Part model, mm, in its own coordinate system. Give positions to 0.01 mm unless a question says otherwise; leave off trailing zeros. Write each loop counter-clockwise with the first axis right and the second up, starting at its lowest first coordinate (ties: lowest second). Pieces come first, ordered by that corner, then holes.
```python
from build123d import *

# Parameters (mm, degrees)
SKETCH_1_W           = 0.6
SKETCH_1_H           = 0.6
EXTRUDE_1_DEPTH      = 2
EXTRUDE_2_DEPTH      = 6
EXTRUDE_2_DEPTH_BACK = 5
SKETCH_2_W           = 0.6
SKETCH_2_H           = 0.6


with BuildPart() as part:
    # 草图1 → 凸台-拉伸1 (new body)
    with BuildSketch(Plane.XY):
        Polygon((-0.762, 1.27), (-1.27, 0.762), (-1.27, -0.762), (-0.762, -1.27), (0.762, -1.27), (1.27, -0.762), (1.778, -1.27), (3.302, -1.27), (3.81, -0.762), (4.318, -1.27), (5.842, -1.27), (6.35, -0.762), (6.35, 0.762), (5.842, 1.27), (4.318, 1.27), (3.81, 0.762), (3.302, 1.27), (1.778, 1.27), (1.27, 0.762), (0.762, 1.27), align=None)
        with Locations((2.54, 0)):
            Rectangle(SKETCH_1_W, SKETCH_1_H, mode=Mode.SUBTRACT)
        Rectangle(SKETCH_1_W, SKETCH_1_H, mode=Mode.SUBTRACT)
        with Locations((5.08, 0)):
            Rectangle(SKETCH_1_W, SKETCH_1_H, mode=Mode.SUBTRACT)
    extrude(amount=EXTRUDE_1_DEPTH)

    # 草图2 → 凸台-拉伸2 (add, two sides: drawn at the far end of the back side and taken through both)
    with BuildSketch(Plane.XY.offset(2).offset(-EXTRUDE_2_DEPTH_BACK)):
        Rectangle(SKETCH_2_W, SKETCH_2_H)
        with Locations((2.54, 0)):
            Rectangle(SKETCH_2_W, SKETCH_2_H)
        with Locations((5.08, 0)):
            Rectangle(SKETCH_2_W, SKETCH_2_H)
    extrude(amount=EXTRUDE_2_DEPTH + EXTRUDE_2_DEPTH_BACK)


solid = part.part
```
1) Saw through at A-A, the plane z = 3.5. Write the cut outline in (x, y), then the cut area to 3 significant figures.
Answers follow:
outline: (-0.3, -0.3) - (0.3, -0.3) - (0.3, 0.3) - (-0.3, 0.3) - close; (2.24, -0.3) - (2.84, -0.3) - (2.84, 0.3) - (2.24, 0.3) - close; (4.78, -0.3) - (5.38, -0.3) - (5.38, 0.3) - (4.78, 0.3) - close
area: 1.08 mm2
2) Saw through at C-C, the plane x = 0. Write the cut outline in (y, z), then the cut area to 3 significant figures.
Answers follow:
outline: (-1.27, 0) - (-0.3, 0) - (-0.3, -3) - (0.3, -3) - (0.3, 0) - (1.27, 0) - (1.27, 2) - (0.3, 2) - (0.3, 8) - (-0.3, 8) - (-0.3, 2) - (-1.27, 2) - close
area: 10.5 mm2
3) Wall check: L1, parallel to X at y = 0.1, z = 2.25; L2, parallel to X at y = -1, z = 1.75; L3, parallel to Z at x = 6, y = -0.6. Give the ranges that are in metal, low to high.
Answers follow:
L1: x = -0.3 to 0.3, 2.24 to 2.84, 4.78 to 5.38
L2: x = -1.03 to 1.03, 1.51 to 3.57, 4.05 to 6.11
L3: z = 0 to 2
4) Saw through at D-D, the plane z = 1.5. Write the cut outline in (x, y).
Answers follow:
outline: (-1.27, -0.76) - (-0.76, -1.27) - (0.76, -1.27) - (1.27, -0.76) - (1.78, -1.27) - (3.3, -1.27) - (3.81, -0.76) - (4.32, -1.27) - (5.84, -1.27) - (6.35, -0.76) - (6.35, 0.76) - (5.84, 1.27) - (4.32, 1.27) - (3.81, 0.76) - (3.3, 1.27) - (1.78, 1.27) - (1.27, 0.76) - (0.76, 1.27) - (-0.76, 1.27) - (-1.27, 0.76) - close
5) Saw through at B-B, the plane y = 1.05. Write the cut outline in (x, z), then the cut area to 3 significant figures.
Answers follow:
outline: (-0.98, 0) - (0.98, 0) - (0.98, 2) - (-0.98, 2) - close; (1.56, 0) - (3.52, 0) - (3.52, 2) - (1.56, 2) - close; (4.1, 0) - (6.06, 0) - (6.06, 2) - (4.1, 2) - close
area: 11.8 mm2
6) Pin check, flat tips, straight feed: pin 1 Ø1 at (x, z) = (0.5, -1) entering from -Y; pin 2 Ø1.3 at (x, y) = (1, 0) entering from -Z; pin 3 Ø0.5 at (x, z) = (0, 4.5) entering from +Y. Stop position of each tip, or through.
Answers follow:
pin 1: stops at y = -0.3
pin 2: stops at z = 0
pin 3: stops at y = 0.3
